Source: CAD feature listing. Evaluate the final solid. Frame: model axes, mm. A direction names the side the tool comes from. Give positions to 0.01 mm unless a question says otherwise; leave off trailing zeros. Write each loop counter-clockwise with the first axis right and the second up, starting at its lowest first coordinate (ties: lowest second). Pieces come first, ordered by that corner, then holes.
```python
from build123d import *

# Parameters (mm, degrees)
F0_W     = 600
F0_H     = 1800
F1_DEPTH = 200
F2_W     = 100
F2_H     = 60
F3_DEPTH = 600
F4_W     = 50
F4_H     = 1600
F5_DEPTH = 100


with BuildPart() as f1:
    # F0 (on Front) → F1 (new body)
    with BuildSketch(Plane.XZ):
        with Locations((300, 900)):
            Rectangle(F0_W, F0_H)
    extrude(amount=F1_DEPTH)

    # F2 (on face) → F3 (join)
    with BuildSketch(Plane.XZ.offset(200)):
        with Locations((50, 30)):
            Rectangle(F2_W, F2_H)
        with Locations((550, 30)):
            Rectangle(F2_W, F2_H)
    extrude(amount=F3_DEPTH)

    # F4 (on face) → F5 (cut)
    with BuildSketch(Plane.XZ.offset(200)):
        with Locations((125, 900)):
            Rectangle(F4_W, F4_H)
        with Locations((475, 900)):
            Rectangle(F4_W, F4_H)
    extrude(amount=-F5_DEPTH, mode=Mode.SUBTRACT)


solid = f1.part
```
1. Access query for faces 4 (the flat face through (500, -151, 889)), 5 (the flat face through (100, -496, 30)), 6 (the flat face through (49, -496, 60)), 7 (the flat face through (0, -161, 829)), 8 (the flat face through (96, -306, 0)). Directions: +Z, -Z, +X, -X, +Y, -Y. A direction counts if a zero-diameter tool reaches every point of the face in a straight line with its end or side. Return the directions, or none.
2. Section query C-C (x = 130.5). Return loops of the section in (y, z), plus the area to 3 significant figures.
3. Line query: probe 1 along X at (y, z) = (-196, 935.5); probe 2 along Y at (x, z) = (228.5, 1471.5); probe 3 along Z at (x, y) = (512, -323). Output: solid intervals per line, ascending.
4. Section query A-A (y = -342.5). Return loops of the section in (x, z).
5. Section query B-B (z = 1452). Return loops of the section in (x, y), plus the area to 3 significant figures.
6. Section query D-D (x = 406.5). Return loops of the section in (y, z), plus the area to 3 significant figures.
7. Pull-direction query (X, two-part tool) for faces 1 (the flat face through (475, -151, 1700)), 2 (the flat face through (549, -800, 30)), 3 (the flat face through (600, -161, 829)); classes: pulls with the +X half, pulls with the -X half, needs draft (parallel to the pull), parting line crosses it, or undercut.
8. Pin query (flat end, axial travel): P1, Ø15, axis at x = 133, z = 592.5, coming from the -Y side; P2, Ø10, axis at x = 102, z = 1278, coming from the -Y side. Return the tip coordinate at first contact, or that it passes through.
The answers:
1. face 4: -Y
1. face 5: +Z, -Z, -Y
1. face 6: +Z, +X, -X, -Y
1. face 7: +Z, -Z, -X, +Y, -Y
1. face 8: -Z, +X, -X, +Y, -Y
2. outline: (-200, 0) - (0, 0) - (0, 1800) - (-200, 1800) - (-200, 1700) - (-100, 1700) - (-100, 100) - (-200, 100) - close
2. area: 200,000 mm2
3. probe 1: x = 0 to 100, 150 to 450, 500 to 600
3. probe 2: y = -200 to 0
3. probe 3: z = 0 to 60
4. outline: (0, 0) - (100, 0) - (100, 60) - (0, 60) - close; (500, 0) - (600, 0) - (600, 60) - (500, 60) - close
5. outline: (0, -200) - (100, -200) - (100, -100) - (150, -100) - (150, -200) - (450, -200) - (450, -100) - (500, -100) - (500, -200) - (600, -200) - (600, 0) - (0, 0) - close
5. area: 110,000 mm2
6. outline: (-200, 0) - (0, 0) - (0, 1800) - (-200, 1800) - close
6. area: 360,000 mm2
7. face 1: undercut
7. face 2: needs draft
7. face 3: pulls with the +X half
8. P1: stops at y = -100
8. P2: stops at y = -200
